```python
from build123d import *

# Parameters (mm, degrees)
SKETCH_1_R      = 14
SKETCH_1_R_2    = 1.5
SKETCH_1_R_3    = 9
SKETCH_1_R_4    = 7.5
EXTRUDE_1_DEPTH = 7
SKETCH_1_3_R    = 9
SKETCH_1_3_R_2  = 7.5
EXTRUDE_2_DEPTH = 9
CHAMFER_1_SIZE  = 0.3
CHAMFER_4_SIZE  = 0.2


with BuildPart() as part:
    # Sketch 1 → Extrude 1 (new body)
    with BuildSketch(Plane(origin=(0, 0, 0), x_dir=(1, 0, 0), z_dir=(0, 1, 0))):
        Circle(SKETCH_1_R)
        with Locations((-11, 0)):
            Circle(SKETCH_1_R_2, mode=Mode.SUBTRACT)
        with Locations((0, -11)):
            Circle(SKETCH_1_R_2, mode=Mode.SUBTRACT)
        with Locations((11, 0)):
            Circle(SKETCH_1_R_2, mode=Mode.SUBTRACT)
        with Locations((0, 11)):
            Circle(SKETCH_1_R_2, mode=Mode.SUBTRACT)
        Circle(SKETCH_1_R_3, mode=Mode.SUBTRACT)
        Circle(SKETCH_1_R_3)
        Circle(SKETCH_1_R_4, mode=Mode.SUBTRACT)
    extrude(amount=EXTRUDE_1_DEPTH)

    # Sketch 1_3 → Extrude 2 (add)
    with BuildSketch(Plane(origin=(0, 0, 0), x_dir=(1, 0, 0), z_dir=(0, 1, 0))):
        Circle(SKETCH_1_3_R)
        Circle(SKETCH_1_3_R_2, mode=Mode.SUBTRACT)
    extrude(amount=EXTRUDE_2_DEPTH)

    # Chamfer 1
    chamfer_1_edges = [part.edges().sort_by_distance(p)[0] for p in [
        (-7.5, 9, 0),
        (-9, 9, 0),
        (-14, 7, 0),
    ]]
    chamfer(chamfer_1_edges, length=CHAMFER_1_SIZE)

    # Chamfer 4
    chamfer_4_edges = [part.edges().sort_by_distance(p)[0] for p in [
        (-14, 0, 0),
    ]]
    chamfer(chamfer_4_edges, length=CHAMFER_4_SIZE)


solid = part.part
```
Geometry check sheet. Reference: the model listing, model coordinates, mm. A direction names the side the tool comes from. Coordinates: 2 decimals unless noted, no trailing zeros. Order: outer loops, then holes, each group sorted by start corner. A loop starts at its lowest first (then second) coordinate and runs counter-clockwise, first axis right, second up. Notation, with made-up numbers: (79, 14) - (109, 14) arc R19 ccw to (109, 29) - close; hole circle Ø4 at (60, -6.5). An arc over 180 degrees is marked (long way). Answer in a Markdown table with one row per item. Add a question column.
1. Access from +Z, -Z, +X, -X, +Y, -Y to the whole of each face (thin tool, end or side, straight path). Record for faces 5 (the face through (6, 0, 6)), 6 (the face through (9, 7, 3)).
2. Section check A-A (x = 0). Enter the section's corners in (y, z).
3. Gauge pin test, flat ends, axial feed: pin 1 Ø1.5 at (x, z) = (11, 7) entering from +Y; pin 2 Ø6 at (x, z) = (-9.5, 7) entering from +Y; pin 3 Ø4 at (x, y) = (-11, 3.5) entering from -Z. Record the tip position at first contact, or that the pin passes through.
4. Section check B-B (y = 5.25). Enter the section's corners in (x, z), plus the area to 3 significant figures.
5. Draft check along Z on faces 1 (the face through (-0.325, 3.451, -9.536)), 2 (the face through (-12.5, 3.45, -0.07)), 3 (the face through (-1.172, 7.838, -8.923)), 4 (the face through (-1, 9, -8)). Enter one of: +Z half, -Z half, draft (parallel to the pull), parting line (faces both ways), or undercut.
6. Material ranges on L1, parallel to X at y = 4.5, z = 0; L2, parallel to X at y = 8.25, z = 0.25, recorded low to high. Write a range as [from, to].
Data:
| question | item | result |
|---|---|---|
| 1 | face 5 | +Z, -Z, +X, -X, -Y |
| 1 | face 6 | +Y |
| 2 | outline | (0, -13.8) - (0.2, -14) - (6.7, -14) - (7, -13.7) - (7, -12.5) - (0, -12.5) - close; (0, -9.5) - (7, -9.5) - (7, -9) - (8.7, -9) - (9, -8.7) - (9, -7.8) - (8.7, -7.5) - (0, -7.5) - close; (0, 7.5) - (8.7, 7.5) - (9, 7.8) - (9, 8.7) - (8.7, 9) - (7, 9) - (7, 9.5) - (0, 9.5) - close; (0, 12.5) - (7, 12.5) - (7, 13.7) - (6.7, 14) - (0.2, 14) - (0, 13.8) - close |
| 3 | pin 1 | stops at y = 7 |
| 3 | pin 2 | stops at y = 8.9 |
| 3 | pin 3 | stops at z = -10.72 |
| 4 | outline | circle Ø28 at (0, 0); hole circle Ø3 at (-11, 0); hole circle Ø15 at (0, 0); hole circle Ø3 at (0, -11); hole circle Ø3 at (0, 11); hole circle Ø3 at (11, 0) |
| 4 | area | 411 mm² |
| 5 | face 1 | undercut |
| 5 | face 2 | undercut |
| 5 | face 3 | parting line |
| 5 | face 4 | draft |
| 6 | L1 | x = [-14, -12.5], [-9.5, -7.5], [7.5, 9.5], [12.5, 14] |
| 6 | L2 | x = [-9, -7.5], [7.5, 9] |
